Answer from the drawing. Dimensions are ordinates in mm from the lowest x, y and z of the part. A direction names the side the tool comes from. Round coordinates to 2 decimals unless told otherwise and drop trailing zeros. Loops run counter-clockwise (first coordinate to the right, second up) from the corner with the lowest first, then second, coordinate; pieces in that order, holes last. Notation, with made-up numbers: (-1.75, -39.5) -> (16.25, -39.5) arc R26 ccw to (16.25, -20.5) -> close; hole circle Ø9 at (14.25, 78). An arc over 180 degrees is marked (long way). One line per question, with ' | ' between items.
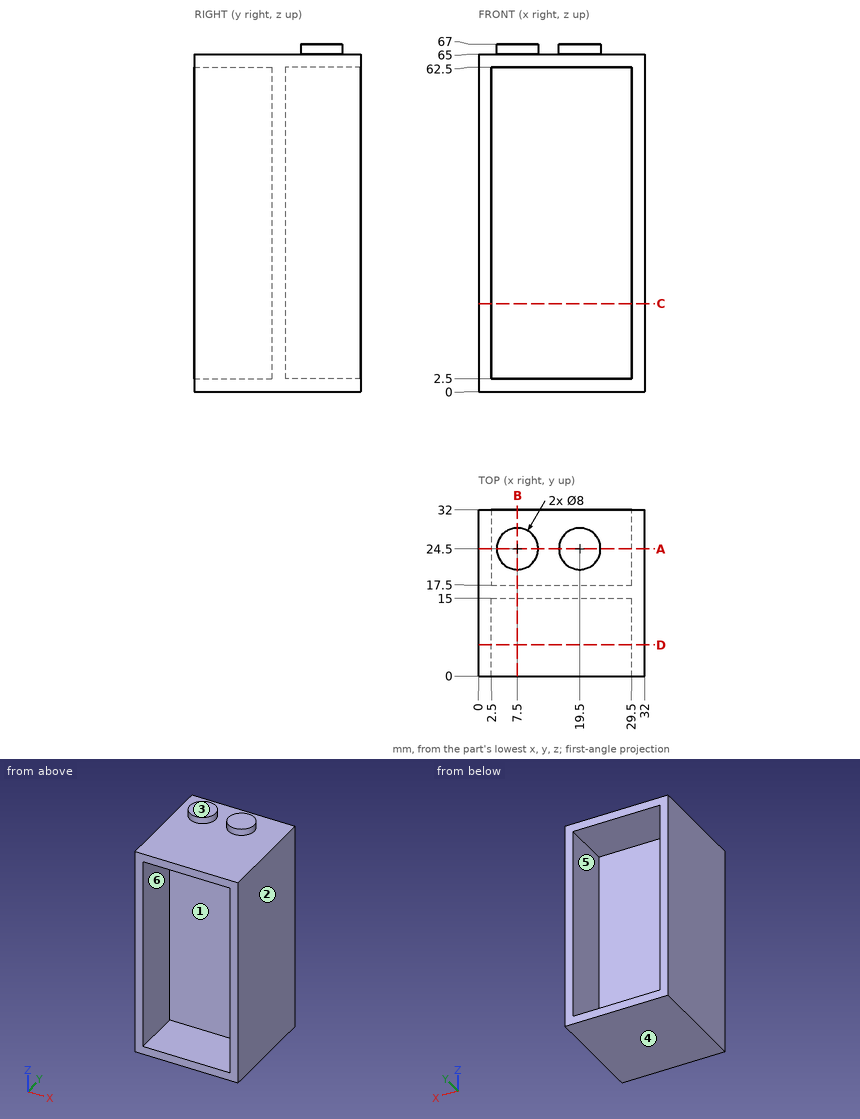
Q1. For a pull along Z with two mould halves and no side action, classify the marked faces 1, 2 and 3 as pulls with the +Z half, pulls with the -Z half, needs draft (parallel to the pull), parting line crosses it, or undercut.
Numbers:
face 1: undercut | face 2: needs draft | face 3: pulls with the +Z half
Q2. A cutting plane is placed at C-C on z = 17. Give the vertices of the cut face in (x, y).
Numbers:
outline: (0, 0) -> (2.5, 0) -> (2.5, 15) -> (29.5, 15) -> (29.5, 0) -> (32, 0) -> (32, 32) -> (29.5, 32) -> (29.5, 17.5) -> (2.5, 17.5) -> (2.5, 32) -> (0, 32) -> close
Q3. A cutting plane is placed at B-B on x = 7.5. Give the vertices of the cut face in (y, z).
Numbers:
outline: (0, 0) -> (32, 0) -> (32, 2.5) -> (17.5, 2.5) -> (17.5, 62.5) -> (32, 62.5) -> (32, 65) -> (28.5, 65) -> (28.5, 67) -> (20.5, 67) -> (20.5, 65) -> (0, 65) -> (0, 62.5) -> (15, 62.5) -> (15, 2.5) -> (0, 2.5) -> close
Q4. For the marked faces 4, 5 and 6, determine the directions among +Z, -Z, +X, -X, +Y, -Y from which every point of the face is accessible in a straight line to the end or side of a thin tool.
Numbers:
face 4: -Z, +X, -X, +Y, -Y | face 5: +Y | face 6: -Y
Q5. A cutting plane is placed at A-A on y = 24.5. Give the vertices of the cut face in (x, z), plus the area to 3 significant figures.
Numbers:
outline: (0, 0) -> (32, 0) -> (32, 65) -> (23.5, 65) -> (23.5, 67) -> (15.5, 67) -> (15.5, 65) -> (11.5, 65) -> (11.5, 67) -> (3.5, 67) -> (3.5, 65) -> (0, 65) -> close; hole (2.5, 2.5) -> (29.5, 2.5) -> (29.5, 62.5) -> (2.5, 62.5) -> close | area: 492 mm^2
Q6. Find the intervals of material crossed by line 1 (Z direction, x = 3.5, y = 23.5); line 2 (X direction, y = 9, z = 44); line 3 (Z direction, x = 19.5, y = 27.5), in increasing order. Write a range as from..to.
Numbers:
line 1: 0..2.5, 62.5..65 | line 2: 0..2.5, 29.5..32 | line 3: 0..2.5, 62.5..67
Q7. A cutting plane is placed at D-D on y = 6. Give the vertices of the cut face in (x, z).
Numbers:
outline: (0, 0) -> (32, 0) -> (32, 65) -> (0, 65) -> close; hole (2.5, 2.5) -> (29.5, 2.5) -> (29.5, 62.5) -> (2.5, 62.5) -> close
Q8. Given pin 1 Ø7.5 at (x, y) = (15, 11) entering from +Z; pin 2 Ø8 at (x, z) = (19, 37) entering from +Y; pin 3 Ø4 at (x, z) = (11, 36) entering from -Y, each flat-ended and moving along its own axis, determine where each tip first touches the part or whether it passes through.
Numbers:
pin 1: z = 65 | pin 2: y = 17.5 | pin 3: y = 15
